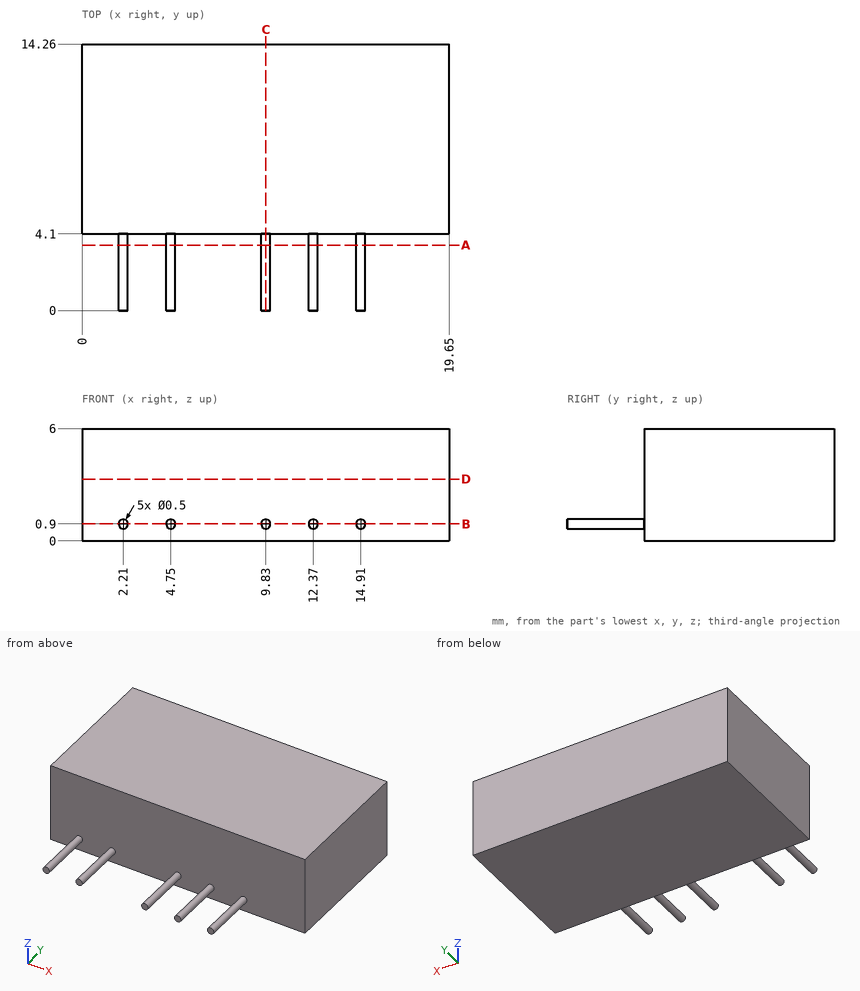
Source: three-view drawing plus pictorial views. Frame: mm from the lowest corner of the part. Give positions to 0.01 mm unless a question says otherwise; leave off trailing zeros. Order: outer loops, then holes, each group sorted by start corner. A loop starts at its lowest first (then second) coordinate and runs counter-clockwise, first axis right, second up. Notation, with made-up numbers: (-7, 89) -> (9, 89) arc R19 ccw to (9, 95) -> close; hole circle Ø11 at (-15.5, 56.25). An arc over 180 degrees is marked (long way). Write each question's results on one line, items separated by ' | '. Start each with the question number.
Item 1: Cut plane A-A on y = 3.5. Return the cut outline in (x, z), then the cut area to 3 significant figures.
Item 2: Cut plane B-B on z = 0.9. Return the cut outline in (x, y), then the cut area to 3 significant figures.
Item 3: Line query: line 1 (Y direction, x = 4.25, z = 3.4); line 2 (X direction, y = 3.75, z = 0.7); line 3 (Z direction, x = 2.25, y = 1). Output: solid intervals per line, ascending.
Item 4: Cut plane D-D on z = 3.3. Return the cut outline in (x, y), then the cut area to 3 significant figures.
Item 5: Cut plane C-C on x = 9.83. Return the cut outline in (y, z).
Established:
1) outline: circle Ø0.5 at (2.21, 0.9); circle Ø0.5 at (4.75, 0.9); circle Ø0.5 at (9.83, 0.9); circle Ø0.5 at (12.37, 0.9); circle Ø0.5 at (14.91, 0.9) | area: 0.982 mm^2
2) outline: (0, 4.1) -> (1.96, 4.1) -> (1.96, 0) -> (2.46, 0) -> (2.46, 4.1) -> (4.5, 4.1) -> (4.5, 0) -> (5, 0) -> (5, 4.1) -> (9.58, 4.1) -> (9.58, 0) -> (10.08, 0) -> (10.08, 4.1) -> (12.12, 4.1) -> (12.12, 0) -> (12.62, 0) -> (12.62, 4.1) -> (14.66, 4.1) -> (14.66, 0) -> (15.16, 0) -> (15.16, 4.1) -> (19.65, 4.1) -> (19.65, 14.26) -> (0, 14.26) -> close | area: 210 mm^2
3) line 1: 4.1 to 14.26 | line 2: 2.06 to 2.36, 4.6 to 4.9, 9.68 to 9.98, 12.22 to 12.52, 14.76 to 15.06 | line 3: 0.65 to 1.15
4) outline: (0, 4.1) -> (19.65, 4.1) -> (19.65, 14.26) -> (0, 14.26) -> close | area: 200 mm^2
5) outline: (0, 0.65) -> (4.1, 0.65) -> (4.1, 0) -> (14.26, 0) -> (14.26, 6) -> (4.1, 6) -> (4.1, 1.15) -> (0, 1.15) -> close
